Design review of the part shown in the three views and the two pictorial views. Dimensions are in mm from the part's minimum x, y and z. Coordinates: 2 decimals unless noted, no trailing zeros. Write each loop counter-clockwise with the first axis right and the second up, starting at its lowest first coordinate (ties: lowest second). Pieces come first, ordered by that corner, then holes. Notation, with made-up numbers: (13.25, 3) - (32.25, 3) arc R30 ccw to (32.25, 39) - close; hole circle Ø3 at (0, 52). An arc over 180 degrees is marked (long way). Return JSON: item names as keys, results as strings. Group by question number.
(1) We need section B-B on x = 16.51. State the section outline as (y, z) points.
(2) To check wall thickness, follow L1, parallel to X at y = 16.5, z = 1.3; L2, parallel to Y at x = 30, z = 0.9. State the ranges of each line that lie inside material, in increasing order. Write a range as from..to.
(3) We need section A-A on y = 24.01. State the section outline as (x, z) points.
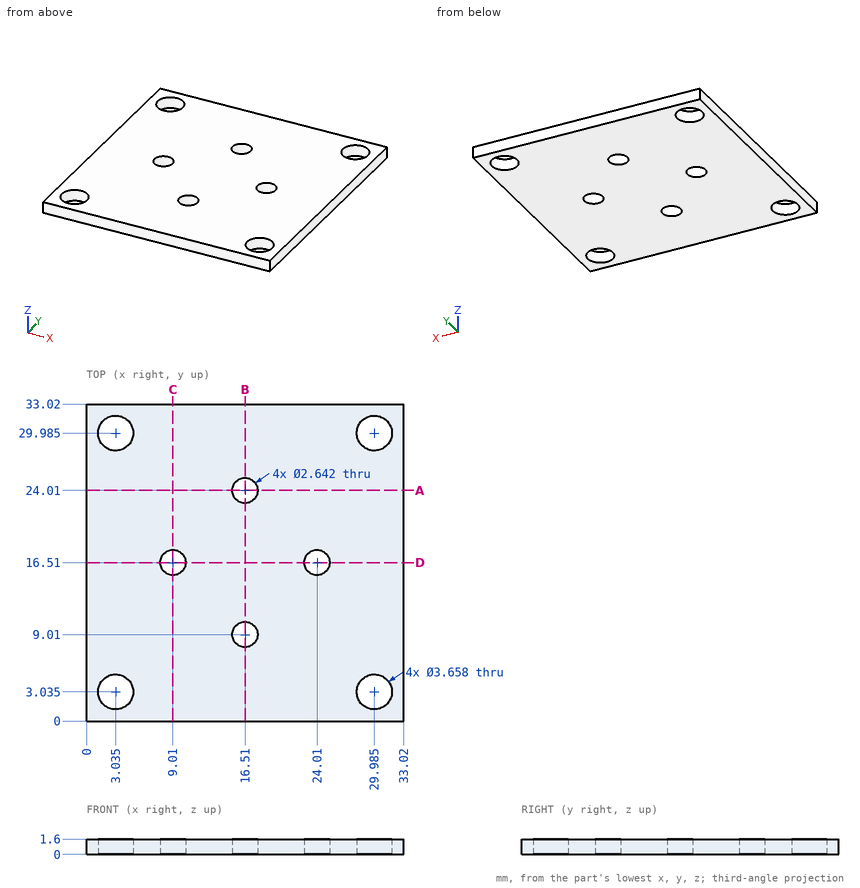
Ans:
{
 "1": {"outline": "(0, 0) - (7.69, 0) - (7.69, 1.6) - (0, 1.6) - close; (10.33, 0) - (22.69, 0) - (22.69, 1.6) - (10.33, 1.6) - close; (25.33, 0) - (33.02, 0) - (33.02, 1.6) - (25.33, 1.6) - close"},
 "2": {"L1": "0..7.69, 10.33..22.69, 25.33..33.02", "L2": "0..1.21, 4.86..28.16, 31.81..33.02"},
 "3": {"outline": "(0, 0) - (15.19, 0) - (15.19, 1.6) - (0, 1.6) - close; (17.83, 0) - (33.02, 0) - (33.02, 1.6) - (17.83, 1.6) - close"}
}
